Read the model definition and answer for the solid it produces. Units are mm, in the model's axes. Face numbers are marked on the shaded views. Give positions to 0.01 mm unless a question says otherwise; leave off trailing zeros. Loops run counter-clockwise (first coordinate to the right, second up) from the corner with the lowest first, then second, coordinate; pieces in that order, holes last.
(1) Straight lines are drawn through the part: probe 1 along Y at (x, z) = (-12.5, 1.9); probe 2 along Y at (x, z) = (19, 3.5); probe 3 along Y at (x, z) = (19, 6.25). For each, find the intervals that lie inside material, in ascending order.
(2) Determine the mould class of the marked faces 1 and 2 for opening direction Y: pulls with the +Y half, pulls with the -Y half, needs draft (parallel to the pull), parting line crosses it, or undercut.
(3) Find section A-A, the plane x = 31.5. Write down the section's boundary in (y, z), then the cut area to 3 significant figures.
(4) Find section D-D, the plane y = -13.5. Write down the section's boundary in (x, z).
(5) Find section C-C, the plane z = 7.5. State how many separate pieces and enclosed holes the cut face has, then the cut area to 3 significant figures.
(6) Each of these flat-tipped pins is pushed along its axis until it touches: P1, Ø4.5, axis at y = -25.5, z = 8.5, coming from the +X side; P2, Ø5, axis at x = 15, y = -4, coming from the +Z side; P3, Ø3, axis at x = 31.5, y = -3.5, coming from the -Z side. Where does it stop, or does it pass through?
(7) Find section B-B, the plane y = -3.5. Write down the section's boundary in (x, z).
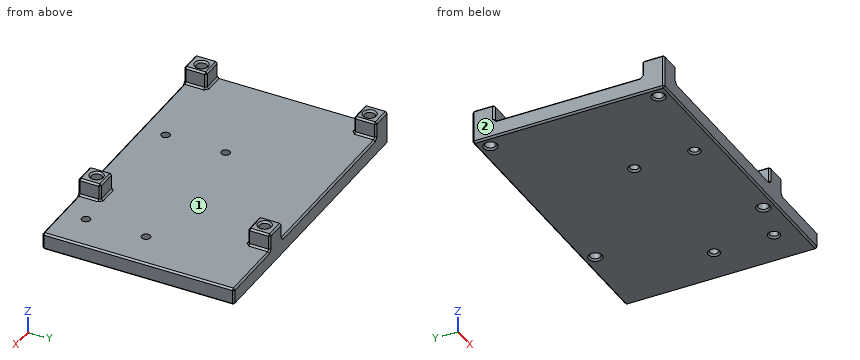
```python
from build123d import *

# Parameters (mm, degrees)
SKETCH_W        = 85
SKETCH_H        = 56
PAD_DEPTH       = 5
SKETCH001_W     = 6.5
SKETCH001_H     = 6.5
PAD001_DEPTH    = 5
SKETCH002_R     = 1.5
POCKET_DEPTH    = 10.001
SKETCH003_R     = 1.25
POCKET001_DEPTH = 10.001
CHAMFER_SIZE    = 0.5


with BuildPart() as part:
    # Sketch (on XY_Plane of Origin) → Pad (new body)
    with BuildSketch(Plane.XY):
        Rectangle(SKETCH_W, SKETCH_H)
    extrude(amount=PAD_DEPTH)

    # Sketch001 (on Face6 of Pad) → Pad001 (join)
    with BuildSketch(Plane.XY.offset(5)):
        with Locations((-39.25, 24.75)):
            Rectangle(SKETCH001_W, SKETCH001_H)
        with Locations((-39.25, -24.75)):
            Rectangle(SKETCH001_W, SKETCH001_H)
        with Locations((19.25, 24.75)):
            Rectangle(SKETCH001_W, SKETCH001_H)
        with Locations((19.25, -24.75)):
            Rectangle(SKETCH001_W, SKETCH001_H)
    extrude(amount=PAD001_DEPTH)

    # Sketch002 (on Face5 of Pad001) → Pocket (cut, through all)
    with BuildSketch(Plane.XY.offset(10)):
        with Locations((-39, 24.5)):
            Circle(SKETCH002_R)
        with Locations((-39, -24.5)):
            Circle(SKETCH002_R)
        with Locations((19, 24.5)):
            Circle(SKETCH002_R)
        with Locations((19, -24.5)):
            Circle(SKETCH002_R)
    extrude(amount=-POCKET_DEPTH, mode=Mode.SUBTRACT)

    # Sketch003 (on Face1 of Pocket) → Pocket001 (cut, through all)
    with BuildSketch(Plane(origin=(0, 0, 0), x_dir=(1, 0, 0), z_dir=(0, 0, -1))):
        with Locations((31.5, 21)):
            Circle(SKETCH003_R)
        with Locations((31.5, 3.5)):
            Circle(SKETCH003_R)
        with Locations((-12.5, 21)):
            Circle(SKETCH003_R)
        with Locations((-12.5, 3.5)):
            Circle(SKETCH003_R)
    extrude(amount=-POCKET001_DEPTH, mode=Mode.SUBTRACT)

    # Chamfer
    chamfer_edges = [part.edges().sort_by_distance(p)[0] for p in [
        (42.5, 28, 2.5),
        (0, 28, 0),
        (-42.5, 28, 5),
        (-39.25, 28, 10),
        (-36, 28, 7.5),
        (-10, 28, 5),
        (16, 28, 7.5),
        (19.25, 28, 10),
        (22.5, 28, 7.5),
        (32.5, 28, 5),
        (-42.5, 0, 0),
        (-42.5, -28, 5),
        (-42.5, -24.75, 10),
        (-42.5, -21.5, 7.5),
        (-42.5, 0, 5),
        (-42.5, 21.5, 7.5),
        (-42.5, 24.75, 10),
        (0, -28, 0),
        (42.5, -28, 2.5),
        (32.5, -28, 5),
        (22.5, -28, 7.5),
        (19.25, -28, 10),
        (16, -28, 7.5),
        (-10, -28, 5),
        (-36, -28, 7.5),
        (-39.25, -28, 10),
        (42.5, 0, 0),
        (42.5, 0, 5),
        (-36, -24.75, 10),
        (-39.25, -21.5, 10),
        (-40.5, -24.5, 10),
        (-39.25, 21.5, 10),
        (-36, 24.75, 10),
        (-40.5, 24.5, 10),
        (16, 24.75, 10),
        (19.25, 21.5, 10),
        (22.5, 24.75, 10),
        (17.5, 24.5, 10),
        (16, -24.75, 10),
        (22.5, -24.75, 10),
        (19.25, -21.5, 10),
        (17.5, -24.5, 10),
        (22.5, -21.5, 7.5),
        (22.5, -24.75, 5),
        (16, -21.5, 7.5),
        (19.25, -21.5, 5),
        (16, -24.75, 5),
        (-36, -21.5, 7.5),
        (-36, -24.75, 5),
        (-39.25, -21.5, 5),
        (-36, 21.5, 7.5),
        (-36, 24.75, 5),
        (-39.25, 21.5, 5),
        (22.5, 21.5, 7.5),
        (22.5, 24.75, 5),
        (16, 21.5, 7.5),
        (19.25, 21.5, 5),
        (16, 24.75, 5),
        (17.5, -24.5, 0),
        (-40.5, -24.5, 0),
        (-13.75, -21, 0),
        (-13.75, -3.5, 0),
        (30.25, -3.5, 0),
        (30.25, -21, 0),
        (17.5, 24.5, 0),
        (-40.5, 24.5, 0),
    ]]
    chamfer(chamfer_edges, length=CHAMFER_SIZE)


solid = part.part
```
Entries:
1. probe 1: y = -28 to -22.25, -19.75 to -4.75, -2.25 to 28
1. probe 2: y = -28 to -26, -23 to 23, 26 to 28
1. probe 3: y = -28 to -26, -23 to -21.5, 21.5 to 23, 26 to 28
2. face 1: undercut
2. face 2: needs draft
3. outline: (-28, 0.5) - (-27.5, 0) - (-22.75, 0) - (-22.25, 0.5) - (-22.25, 5) - (-27.5, 5) - (-28, 4.5) - close; (-19.75, 0.5) - (-19.25, 0) - (-5.25, 0) - (-4.75, 0.5) - (-4.75, 5) - (-19.75, 5) - close; (-2.25, 0.5) - (-1.75, 0) - (27.5, 0) - (28, 0.5) - (28, 4.5) - (27.5, 5) - (-2.25, 5) - close
3. area: 254 mm2
4. outline: (-42.5, 0.5) - (-42, 0) - (42, 0) - (42.5, 0.5) - (42.5, 4.5) - (42, 5) - (-42, 5) - (-42.5, 4.5) - close
5. separate pieces: 4
5. enclosed holes: 4
5. area: 139 mm2
6. P1: stops at x = 22.5
6. P2: stops at z = 5
6. P3: stops at z = 0.25
7. outline: (-42.5, 0.5) - (-42, 0) - (-14.25, 0) - (-13.75, 0.5) - (-13.75, 5) - (-42, 5) - (-42.5, 4.5) - close; (-11.25, 0.5) - (-10.75, 0) - (29.75, 0) - (30.25, 0.5) - (30.25, 5) - (-11.25, 5) - close; (32.75, 0.5) - (33.25, 0) - (42, 0) - (42.5, 0.5) - (42.5, 4.5) - (42, 5) - (32.75, 5) - close
